Autodesk Inventor part; units mm, degrees
ref_plane "YZ Plane" through (0, 0, 0) normal (1, 0, 0) x (0, 1, 0)
ref_plane "XZ Plane" through (0, 0, 0) normal (0, 1, 0) x (-1, 0, 0)
ref_plane "XY Plane" through (0, 0, 0) normal (0, 0, 1) x (1, 0, 0)
sketch "Sketch1" plane through (0, 0, 0) normal (0, 1, 0) x (-1, 0, 0)
  line L0 (-47.625, 57.15) -> (47.625, 57.15)
  line L1 (47.625, 57.15) -> (47.625, -57.15)
  line L2 (47.625, -57.15) -> (-47.625, -57.15)
  line L3 (-47.625, -57.15) -> (-47.625, 57.15)
  line L4 (-47.625, 57.15) -> (47.625, -57.15) construction
  line L5 (47.625, 57.15) -> (-47.625, -57.15) construction
  point P0 (0, 0)
  dimension "d0" = 114.3
  dimension "d1" = 95.25
extrude "Extrusion1" add sketch "Sketch1" along normal blind 41.275
sketch "Sketch2" plane through (0, 41.275, 0) normal (0, 1, 0) x (1, 0, 0)
  line L0 (28.575, -44.45) -> (-28.575, -44.45)
  line L1 (-34.925, -38.1) -> (-34.925, 38.1)
  line L2 (-28.575, 44.45) -> (28.575, 44.45)
  line L3 (34.925, 38.1) -> (34.925, -38.1)
  line L4 (34.925, -44.45) -> (-34.925, 44.45) construction
  line L5 (-34.925, -44.45) -> (34.925, 44.45) construction
  arc A0 (-34.925, -38.1) -> (-28.575, -44.45) centre (-28.575, -38.1) ccw
  arc A1 (-28.575, 44.45) -> (-34.925, 38.1) centre (-28.575, 38.1) ccw
  arc A2 (34.925, 38.1) -> (28.575, 44.45) centre (28.575, 38.1) ccw
  arc A3 (28.575, -44.45) -> (34.925, -38.1) centre (28.575, -38.1) ccw
  line L6 (-47.625, 57.15) -> (-47.625, -57.15)
  line L7 (47.625, 57.15) -> (-47.625, 57.15)
  point P0 (0, 0)
  dimension "d6" = 6.35
  dimension "d25" = 12.7
  dimension "d26" = 12.7
extrude "Extrusion2" add sketch "Sketch2" along normal blind 25.4
fillet "Fillet1" radius 3.175 8 edges at (33.0651, 66.675, 42.5901) (34.925, 66.675, 0) (33.0651, 66.675, -42.5901) (0, 66.675, -44.45) (-33.0651, 66.675, -42.5901) (-34.925, 66.675, 0) (-33.0651, 66.675, 42.5901) (0, 66.675, 44.45)
hole "Hole1" at (38.1, 41.275, 47.625) direction (0, -1, 0) diameter 6.35 end through all
pattern_linear "Rectangular Pattern1" count 2 spacing 95.25 along (0, 0, -1) count 2 spacing 76.2 along (-1, 0, 0) of "Hole1"
sketch "Sketch3" plane through (0, 0, 0) normal (0, -1, 0) x (1, 0, 0)
  line L0 (-28.575, -44.45) -> (28.575, -44.45)
  line L1 (34.925, -38.1) -> (34.925, 38.1)
  line L2 (28.575, 44.45) -> (-28.575, 44.45)
  line L3 (-34.925, 38.1) -> (-34.925, -38.1)
  line L4 (-34.925, -44.45) -> (34.925, 44.45) construction
  line L5 (34.925, -44.45) -> (-34.925, 44.45) construction
  line L6 (47.625, 57.15) -> (-47.625, 57.15)
  line L7 (47.625, -57.15) -> (47.625, 57.15)
  arc A0 (-28.575, 44.45) -> (-34.925, 38.1) centre (-28.575, 38.1) ccw
  arc A1 (34.925, 38.1) -> (28.575, 44.45) centre (28.575, 38.1) ccw
  arc A2 (28.575, -44.45) -> (34.925, -38.1) centre (28.575, -38.1) ccw
  arc A3 (-34.925, -38.1) -> (-28.575, -44.45) centre (-28.575, -38.1) ccw
  point P0 (0, 0)
  dimension "d27" = 12.7
  dimension "d28" = 12.7
  dimension "d29" = 6.35
extrude "Extrusion3" add sketch "Sketch3" along normal blind 25.4
fillet "Fillet2" radius 3.175 8 edges at (-33.0651, -25.4, 42.5901) (-34.925, -25.4, 0) (-33.0651, -25.4, -42.5901) (0, -25.4, -44.45) (33.0651, -25.4, -42.5901) (34.925, -25.4, 0) (33.0651, -25.4, 42.5901) (0, -25.4, 44.45)
properties part number "xmfr power" material "Iron, Malleable"
Design review of the part built by this model. Coordinates are the model's own, in mm. A direction names the side the tool comes from. Give positions to 0.01 mm unless a question says otherwise; leave off trailing zeros. Write each loop counter-clockwise with the first axis right and the second up, starting at its lowest first coordinate (ties: lowest second). Pieces come first, ordered by that corner, then holes. Notation, with made-up numbers: (-17, 53) - (23, 53) arc R31 cw to (23, 88) - close; hole circle Ø10 at (88, 5). An arc over 180 degrees is marked (long way). Return JSON: item names as keys, results as strings. Group by question number.
(1) Machinability: for faces 4 (the flat face through (43, 0, 1)), 5 (the cylindrical face through (33.114, 52.232, 42.54)), 6 (the cylindrical face through (33.015, -10.957, 42.639)), which of the approach directions +Z, -Z, +X, -X, +Y, -Y give a long, thin tool a straight path to every point of the face, cutting with its end or side? Answer none if there is none.
(2) To check wall thickness, follow probe 1 along Z at (x, y) = (-38.1, 29); probe 2 along X at (y, z) = (29, -46) (3 decimals); probe 3 along X at (y, z) = (-11, 24) (3 decimals). State the ranges of each line that lie inside material, in increasing order.
(3) Insertion check: pin 1 (4 mm diameter, centred on y = -11.5, z = 35, fed in from -X) (3 decimals); pin 2 (6 mm diameter, centred on x = 31.5, y = -6.5, fed in from -Z); pin 3 (2 mm diameter, centred on y = -5, z = 29.5, fed in from +X) (3 decimals). Each pin has a flat end and moves straight along its axis. Give the tip position at first contact, or say it passes through.
(4) We need section B-B, the plane y = 56. Give the boundary of the cut face in (x, z) (3 decimals), then the cut area to 3 significant figures.
(5) We need section A-A, the plane x = -38.1. Give the boundary of the cut face in (y, z) (3 decimals), then the cut area to 3 significant figures.
(6) We need section C-C, the plane x = -23. Give the boundary of the cut face in (y, z) (3 decimals).
(7) We need section D-D, the plane z = 31.5. Give the boundary of the cut face in (x, y) (3 decimals), then the cut area to 3 significant figures.
(8) Mouldability with a two-part tool opening along Z and no side actions: class faces 1 (the flat face through (-34.925, -11, 1)), 2 (the cylindrical face through (-0.4, -24.49, 43.5)), 3 (the cylindrical face through (-39.054, 20.349, -44.597)) as +Z half, -Z half, draft (parallel to the pull), parting line (faces both ways), or undercut.
Reported:
{
 "1": {"face 4": "-Y", "face 5": "+Z, +X, +Y", "face 6": "+Z, +X, -Y"},
 "2": {"probe 1": "z = -57.15 to -50.8, -44.45 to 44.45, 50.8 to 57.15", "probe 2": "x = -47.625 to -40.828, -35.372 to 35.372, 40.828 to 47.625", "probe 3": "x = -34.925 to 34.925"},
 "3": {"pin 1": "stops at x = -34.925", "pin 2": "stops at z = -44.45", "pin 3": "stops at x = 34.925"},
 "4": {"outline": "(-34.925, -38.1) arc R6.35 ccw to (-28.575, -44.45) - (28.575, -44.45) arc R6.35 ccw to (34.925, -38.1) - (34.925, 38.1) arc R6.35 ccw to (28.575, 44.45) - (-28.575, 44.45) arc R6.35 ccw to (-34.925, 38.1) - close", "area": "6,180 mm2"},
 "5": {"outline": "(0, -57.15) - (41.275, -57.15) - (41.275, -50.8) - (0, -50.8) - close; (0, -44.45) - (41.275, -44.45) - (41.275, 44.45) - (0, 44.45) - close; (0, 50.8) - (41.275, 50.8) - (41.275, 57.15) - (0, 57.15) - close", "area": "4,190 mm2"},
 "6": {"outline": "(-25.4, -41.275) arc R3.175 ccw to (-22.225, -44.45) - (0, -44.45) - (0, -57.15) - (41.275, -57.15) - (41.275, -44.45) - (63.5, -44.45) arc R3.175 ccw to (66.675, -41.275) - (66.675, 41.275) arc R3.175 ccw to (63.5, 44.45) - (41.275, 44.45) - (41.275, 57.15) - (0, 57.15) - (0, 44.45) - (-22.225, 44.45) arc R3.175 ccw to (-25.4, 41.275) - close"},
 "7": {"outline": "(-47.625, 0) - (-34.925, 0) - (-34.925, -22.225) arc R3.175 ccw to (-31.75, -25.4) - (31.75, -25.4) arc R3.175 ccw to (34.925, -22.225) - (34.925, 0) - (47.625, 0) - (47.625, 41.275) - (34.925, 41.275) - (34.925, 63.5) arc R3.175 ccw to (31.75, 66.675) - (-31.75, 66.675) arc R3.175 ccw to (-34.925, 63.5) - (-34.925, 41.275) - (-47.625, 41.275) - close", "area": "7,470 mm2"},
 "8": {"face 1": "draft", "face 2": "+Z half", "face 3": "undercut"}
}
